The model under review builds one solid part; all positions refer to its coordinate system, in mm. Face numbers are marked on the shaded views. A direction names the side the tool comes from. Give positions to 0.01 mm unless a question says otherwise; leave off trailing zeros. Write each loop counter-clockwise with the first axis right and the second up, starting at its lowest first coordinate (ties: lowest second). Pieces come first, ordered by that corner, then holes.
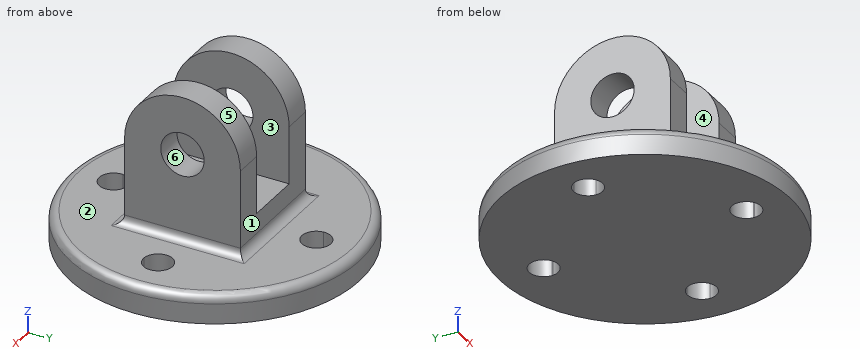
from build123d import *

# Parameters (mm, degrees)
F0_R      = 63.5
F1_DEPTH  = 6.35
F2_W      = 50.8
F2_H      = 50.8
F3_DEPTH  = 76.2
F4_W      = 25.4
F4_H      = 63.5
F5_DEPTH  = 88.901
F6_R      = 9.525
F8_DEPTH  = 88.901
F9_DEPTH  = 88.901
F11_DEPTH = 12.701
F12_R     = 3.81


with BuildPart() as f1:
    # F0 (on Top) → F1 (new body, symmetric)
    with BuildSketch(Plane.XY):
        Circle(F0_R)
    extrude(amount=F1_DEPTH, both=True)

    # F2 (on face) → F3 (join)
    with BuildSketch(Plane.XY.offset(6.35)):
        Rectangle(F2_W, F2_H)
    extrude(amount=F3_DEPTH)

    # F4 (on face) → F5 (cut, through all)
    with BuildSketch(Plane.XZ.offset(25.4)):
        with Locations((0, 50.8)):
            Rectangle(F4_W, F4_H)
    extrude(amount=-F5_DEPTH, mode=Mode.SUBTRACT)

    # F6 (on face) → F8 (cut, through all)
    with BuildSketch(Plane.YZ.offset(25.4)):
        with Locations((0, 44.45)):
            Circle(F6_R)
    extrude(amount=-F8_DEPTH, mode=Mode.SUBTRACT)

    # F7 (on face) → F9 (cut, through all)
    with BuildSketch(Plane.YZ.offset(25.4)):
        with BuildLine():
            ThreePointArc((-25.4, 44.45), (0, 69.85), (25.4, 44.45))
            Line((25.4, 44.45), (25.4, 82.55))
            Line((25.4, 82.55), (-25.4, 82.55))
            Line((-25.4, 82.55), (-25.4, 44.45))
        make_face()
    extrude(amount=-F9_DEPTH, mode=Mode.SUBTRACT)

    # F10 (on face) → F11 (cut, through all)
    with BuildSketch(Plane.XY.offset(6.35)):
        with BuildLine():
            ThreePointArc((-43.9964285714, -6.3337803056), (-44.45, 0), (-43.9964285714, 6.3337803056))
            ThreePointArc((-43.9964285714, 6.3337803056), (-50.8, 0), (-43.9964285714, -6.3337803056))
        make_face()
        with BuildLine():
            ThreePointArc((-38.1, 0), (-39.8022759026, 4.3267956636), (-43.9964285714, 6.3337803056))
            ThreePointArc((-43.9964285714, 6.3337803056), (-44.45, 0), (-43.9964285714, -6.3337803056))
            ThreePointArc((-43.9964285714, -6.3337803056), (-39.8022759026, -4.3267956636), (-38.1, 0))
        make_face()
        with BuildLine():
            ThreePointArc((-6.3337803056, 43.9964285714), (0, 38.1), (6.3337803056, 43.9964285714))
            ThreePointArc((6.3337803056, 43.9964285714), (0, 44.45), (-6.3337803056, 43.9964285714))
        make_face()
        with BuildLine():
            ThreePointArc((-6.3337803056, 43.9964285714), (0, 44.45), (6.3337803056, 43.9964285714))
            ThreePointArc((6.3337803056, 43.9964285714), (6.3459437809, 44.2230693282), (6.35, 44.45))
            ThreePointArc((6.35, 44.45), (-0.2269306718, 50.7959437809), (-6.3337803056, 43.9964285714))
        make_face()
        with BuildLine():
            ThreePointArc((43.9964285714, -6.3337803056), (44.336462139, -3.175), (44.45, 0))
            ThreePointArc((44.45, 0), (44.336462139, 3.175), (43.9964285714, 6.3337803056))
            ThreePointArc((43.9964285714, 6.3337803056), (38.1, 0), (43.9964285714, -6.3337803056))
        make_face()
        with BuildLine():
            ThreePointArc((43.9964285714, 6.3337803056), (44.336462139, 3.175), (44.45, 0))
            ThreePointArc((44.45, 0), (44.336462139, -3.175), (43.9964285714, -6.3337803056))
            ThreePointArc((43.9964285714, -6.3337803056), (48.7767956636, -4.6477240974), (50.8, 0))
            ThreePointArc((50.8, 0), (48.7767956636, 4.6477240974), (43.9964285714, 6.3337803056))
        make_face()
        with BuildLine():
            ThreePointArc((-6.3337803056, -43.9964285714), (0, -44.45), (6.3337803056, -43.9964285714))
            ThreePointArc((6.3337803056, -43.9964285714), (0, -38.1), (-6.3337803056, -43.9964285714))
        make_face()
        with BuildLine():
            ThreePointArc((6.35, -44.45), (6.3459437809, -44.2230693282), (6.3337803056, -43.9964285714))
            ThreePointArc((6.3337803056, -43.9964285714), (0, -44.45), (-6.3337803056, -43.9964285714))
            ThreePointArc((-6.3337803056, -43.9964285714), (-0.2269306718, -50.7959437809), (6.35, -44.45))
        make_face()
    extrude(amount=-F11_DEPTH, mode=Mode.SUBTRACT)

    # F12
    f12_edges = [f1.edges().sort_by_distance(p)[0] for p in [
        (-63.5, 0, 6.35),
        (25.4, 0, 6.35),
        (0, -25.4, 6.35),
        (-25.4, 0, 6.35),
        (0, 25.4, 6.35),
    ]]
    fillet(f12_edges, radius=F12_R)


solid = f1.part
1) The part is to be moulded in two halves that separate along Z. For the marked faces 4, 5 and 6, say which applies: +Z half, -Z half, draft (parallel to the pull), parting line (faces both ways), or undercut.
2) Tool access review of the marked faces 1, 2 and 3: name each direction out of +Z, -Z, +X, -X, +Y, -Y from which nothing blocks a thin tool from reaching the whole face with its end or side.
3) To check wall thickness, follow probe 1 along Z at (x, y) = (17.5, 0) (3 decimals); probe 2 along X at (y, z) = (5.5, 62.5); probe 3 along Y at (x, z) = (21, 44). State the ranges of each line that lie inside material, in increasing order.
4) Consider section B-B, the plane x = 0. Give the boundary of the cut face in (y, z).
5) Consider section A-A, the plane z = -0.5. Give the boundary of the cut face in (x, y).
6) Insertion check: pin 1 (2 mm diameter, centred on x = 23.5, z = 6.5, fed in from +Y); pin 2 (1 mm diameter, centred on x = 9.5, y = 12, fed in from +Z); pin 3 (12 mm diameter, centred on x = 32.5, y = 50.5, fed in from +Z); pin 4 (11.5 mm diameter, centred on y = 0, z = 44.45, fed in from +X). Each pin has a flat end and moves straight along its axis. Give the tip position at first contact, or say it passes through.
7) Consider section C-C, the plane z = 48.5. Give the boundary of the cut face in (x, y), then the cut area to 3 significant figures.
Answer block:
1. face 4: draft
1. face 5: +Z half
1. face 6: undercut
2. face 1: +Z, +X, -X, +Y
2. face 2: +Z
2. face 3: +Z, +Y, -Y
3. probe 1: z = -6.35 to 34.925, 53.975 to 69.85
3. probe 2: x = -25.4 to -12.7, 12.7 to 25.4
3. probe 3: y = -25.4 to -9.51, 9.51 to 25.4
4. outline: (-63.5, -6.35) - (-50.8, -6.35) - (-50.8, 6.35) - (-59.69, 6.35) arc R3.81 ccw to (-63.5, 2.54) - close; (-38.1, -6.35) - (38.1, -6.35) - (38.1, 6.35) - (29.21, 6.35) arc R3.81 cw to (25.4, 10.16) - (25.4, 19.05) - (-25.4, 19.05) - (-25.4, 10.16) arc R3.81 cw to (-29.21, 6.35) - (-38.1, 6.35) - close; (50.8, -6.35) - (63.5, -6.35) - (63.5, 2.54) arc R3.81 ccw to (59.69, 6.35) - (50.8, 6.35) - close
5. outline: circle Ø127 at (0, 0); hole circle Ø12.7 at (-44.45, 0); hole circle Ø12.7 at (0, -44.45); hole circle Ø12.7 at (0, 44.45); hole circle Ø12.7 at (44.45, 0)
6. pin 1: stops at y = 57.53
6. pin 2: stops at z = 19.05
6. pin 3: stops at z = 6.35
6. pin 4: passes through
7. outline: (-25.4, -25.08) - (-12.7, -25.08) - (-12.7, -8.62) - (-25.4, -8.62) - close; (-25.4, 8.62) - (-12.7, 8.62) - (-12.7, 25.08) - (-25.4, 25.08) - close; (12.7, -25.08) - (25.4, -25.08) - (25.4, -8.62) - (12.7, -8.62) - close; (12.7, 8.62) - (25.4, 8.62) - (25.4, 25.08) - (12.7, 25.08) - close
7. area: 836 mm2
